Here's how the part is built. I have some questions about the finished solid (model axes, mm). Round coordinates to 2 decimals unless told otherwise and drop trailing zeros.
Autodesk Fusion 360 part; units mm, degrees
sketch "Skizze1" plane through (0, 0, 0) normal (0, 1, 0) x (1, 0, 0)
  line L0 (0, 107.5) -> (0, -107.5)
  line L1 (50.4279, -19.4927) -> (65, -18.9838)
  line L2 (50.4279, -19.4927) -> (50.0091, -7.5)
  line L3 (50.0091, -7.5) -> (65, -6.9765)
  line L4 (0, 0) -> (59.8475, 0) construction
  spline S0 degree 5 poles (0, -107.5) (6.9963, -107.5) (19.7475, -106.2356) (35.1536, -100.5492) (49.2456, -86.624) (59.4624, -63.5268) (63.6472, -44.237) (65.0113, -30.9473) (65.1348, -22.8452) (65, -18.9838) knots 0 0 0 0 0 0 0.2 0.4 0.6 0.8 1 1 1 1 1 1
  line L5 (65.2619, -26.4838) -> (64.7381, -11.4838)
  line L6 (-12.5, -107.5) -> (12.5, -107.5)
  spline S1 degree 5 poles (0, 107.5) (3.4735, 107.5) (10.463, 106.2697) (21.0748, 100.7368) (35.1986, 86.9145) (51.0909, 61.8673) (60.389, 37.1064) (64.1612, 16.0697) (65, 0.897) (65, -6.9765) knots 0 0 0 0 0 0 0.2 0.4 0.6 0.8 1 1 1 1 1 1
  line L7 (-7.5, 107.5) -> (7.5, 107.5)
  line L8 (65, 13.0235) -> (65, -26.9765)
  dimension "d1" = 215
  dimension "d2" = 107.5
  dimension "d4" = 65
  dimension "d5" = 15
  dimension "d7" = 12
  dimension "d8" = 15
  dimension "d9" = 25
  dimension "d10" = 40
  dimension "d11" = 15
  dimension "d12" = 100
  dimension "d13" = 2
extrude "Extrusion1" add sketch "Skizze1" along normal blind 1.5 contours L0 L1 L2 L3 S0 S1 L8 | S0 L8
sketch "Skizze2" plane through (0, 1.5, 0) normal (0, 1, 0) x (-1, 0, 0)
  spline S0 degree 5 poles (0, 107.5) (-6.9963, 107.5) (-19.7475, 106.2356) (-35.1536, 100.5492) (-49.2456, 86.624) (-59.4624, 63.5268) (-63.6472, 44.237) (-65.0113, 30.9473) (-65.1348, 22.8452) (-65, 18.9838) knots 0 0 0 0 0 0 0.2 0.4 0.6 0.8 1 1 1 1 1 1
  line L0 (-65, 18.9838) -> (-50.4279, 19.4927)
  line L1 (-50.4279, 19.4927) -> (-50.0091, 7.5)
  line L2 (-50.0091, 7.5) -> (-65, 6.9765)
  spline S1 degree 5 poles (-65, 6.9765) (-65, -0.897) (-64.1612, -16.0697) (-60.389, -37.1064) (-51.0909, -61.8673) (-35.1986, -86.9145) (-21.0748, -100.7368) (-10.463, -106.2697) (-3.4735, -107.5) (0, -107.5) knots -1 -1 -1 -1 -1 -1 -0.8 -0.6 -0.4 -0.2 0 0 0 0 0 0
  line L3 (0, -107.5) -> (0, 107.5)
  line L4 (-10, -105.5059) -> (-10, 106.9256) construction
  line L5 (-64.7198, -3.0198) -> (0, -0.7597) construction
  line L6 (-64.8519, 28.9951) -> (0, 31.2598) construction
  circle A0 centre (-27.5, -19.2307) radius 17.5
  circle A1 centre (-22.5, -54.2307) radius 12.5
  circle A2 centre (-17.5, -79.2307) radius 7.5
  circle A3 centre (-27.5, 47.8101) radius 17.5
  circle A4 centre (-21, 82.8101) radius 11
  dimension "d16" = 10
  dimension "d17" = 10
  dimension "d18" = 10
  dimension "d19" = 35
  dimension "d20" = 25
  dimension "d21" = 35
  dimension "d22" = 15
  dimension "d23" = 25
  dimension "d24" = 35
  dimension "d25" = 35
  dimension "d28" = 22
extrude "Extrusion2" cut sketch "Skizze2" against normal blind 5 contours A0 | A1 | A2 | A3 | A4
equation "d2 = d1 / 2"
equation "d18 = d17"
1) I need wall thicknesses on line 1 (Z direction, x = 21, y = 0.7); line 2 (Z direction, x = 32.5, y = 1.05); line 3 (Z direction, x = 17.5, y = 0.8). Which ranges of each line are inside material? Lowest first, please.
2) I'm going to push a flat-ended pin straight in: pin 1 (19.5 mm diameter, centred on x = 17.5, z = -79.23, fed in from +Y). Where does the tip first touch, or does it pass through?
3) If we section it at A-A (x = 27.5): Give the number of separate pieces and of enclosed holes in the cut face, plus the area to 3 significant figures.
4) We'd pull the mould along X, two halves only. Please class faces 1 (the flat face through (32, 0, -2)), 2 (the cylindrical face through (40.398, 0.76, -7.403)), 3 (the cylindrical face through (41.387, 0.76, 37.162)): +X half, -X half, draft (parallel to the pull), parting line (faces both ways), or undercut.
Solutions:
1. line 1: z = -98.99 to -85.86, -72.6 to -66.64, -41.82 to -35.48, -2.98 to 31.56, 64.06 to 71.81, 93.81 to 104.61
1. line 2: z = -87.71 to -61.73, -46.73 to -36, -2.46 to 31.04, 64.58 to 99.41
1. line 3: z = -101.53 to -86.73, -71.73 to -65.69, -42.77 to -33.59, -4.87 to 33.45, 62.17 to 72.38, 93.24 to 105.58
2. pin 1: stops at y = 1.5
3. separate pieces: 5
3. enclosed holes: 0
3. area: 127 mm2
4. face 1: draft
4. face 2: undercut
4. face 3: undercut
